```python
from build123d import *

# Parameters (mm, degrees)
SKETCH1_R               = 1.5
BOSS_EXTRUDE1_DEPTH     = 5
BOSS_EXTRUDE2_DEPTH     = 40
CUT_EXTRUDE1_DEPTH      = 91.434261951
BOSS_EXTRUDE3_START     = -5
BOSS_EXTRUDE3_OUTLINE_R = 2
BOSS_EXTRUDE3_DEPTH     = 5
CUT_EXTRUDE2_START      = -10
CUT_EXTRUDE2_DEPTH      = 10


# Read off the part's stored shape, not the designer's step: Boss-Extrude3
with BuildPart() as part:
    # Sketch1 → Boss-Extrude1 (new body)
    with BuildSketch(Plane(origin=(0, 0, 0), x_dir=(1, 0, 0), z_dir=(0, 1, 0))):
        with BuildLine():
            Line((-57.5, 45.38652637), (-44.5, -53.358277095))
            ThreePointArc((-44.5, -53.358277095), (0, -50.5), (44.5, -53.358277095))
            Line((44.5, -53.358277095), (57.5, 45.38652637))
            ThreePointArc((57.5, 45.38652637), (0, 51), (-57.5, 45.38652637))
        make_face()
        with Locations(Location((-5, 47.5, 0), (0, 0, 270))):
            Circle(SKETCH1_R, mode=Mode.SUBTRACT)
        with Locations(Location((-5, -47.5, 0), (0, 0, 270))):
            Circle(SKETCH1_R, mode=Mode.SUBTRACT)
        with Locations(Location((5, -47.5, 0), (0, 0, 90))):
            Circle(SKETCH1_R, mode=Mode.SUBTRACT)
        with Locations(Location((5, 47.5, 0), (0, 0, 90))):
            Circle(SKETCH1_R, mode=Mode.SUBTRACT)
    extrude(amount=BOSS_EXTRUDE1_DEPTH)

    # Sketch2 → Boss-Extrude2 (add)
    with BuildSketch(Plane(origin=(0, 5, 0), x_dir=(1, 0, 0), z_dir=(0, 1, 0))):
        with BuildLine():
            Line((-26.368366328, 19.603975201), (-20.985908119, -21.279853883))
            ThreePointArc((-20.985908119, -21.279853883), (-20.109118271, -22.872956361), (-18.384839881, -23.450537503))
            ThreePointArc((-18.384839881, -23.450537503), (0, -23), (18.384839881, -23.450537503))
            ThreePointArc((18.384839881, -23.450537503), (20.109118271, -22.872956361), (20.985908119, -21.279853883))
            Line((20.985908119, -21.279853883), (26.368366328, 19.603975201))
            ThreePointArc((26.368366328, 19.603975201), (25.841207036, 21.492926829), (24.11319073, 22.420285883))
            ThreePointArc((24.11319073, 22.420285883), (0, 23.5), (-24.11319073, 22.420285883))
            ThreePointArc((-24.11319073, 22.420285883), (-25.841207036, 21.492926829), (-26.368366328, 19.603975201))
        make_face()
    extrude(amount=BOSS_EXTRUDE2_DEPTH)

    # Sketch3 → Cut-Extrude1 (cut, through all)
    with BuildSketch(Plane(origin=(0, 0, 0), x_dir=(1, 0, 0), z_dir=(0, 1, 0))):
        with BuildLine():
            Line((-21.18897611, 19.181297446), (-16.295136113, -17.99110784))
            ThreePointArc((-16.295136113, -17.99110784), (0, -17.643611739), (16.295136113, -17.99110784))
            Line((16.295136113, -17.99110784), (21.18897611, 19.181297446))
            ThreePointArc((21.18897611, 19.181297446), (0, 19.717805469), (-21.18897611, 19.181297446))
        make_face()
    extrude(amount=CUT_EXTRUDE1_DEPTH, mode=Mode.SUBTRACT)

    # Boss-Extrude3 outline → Boss-Extrude3 (add)
    # profile 1 of 4: a face of its own
    with BuildSketch(Plane.XZ.offset(BOSS_EXTRUDE3_START)):
        with BuildLine():
            Line((-44.496886412, -57.390761561), (-40.51552272, -48.226360981))
            ThreePointArc((-40.51552272, -48.226360981), (-49.028326901, -46.92944202), (-57.5, -45.38652637))
            Line((-57.5, -45.38652637), (-55.934374164, -55.884987732))
            ThreePointArc((-55.934374164, -55.884987732), (-50.783157153, -60.948669168), (-44.496886412, -57.390761561))
        make_face()
        with Locations((-50, -55)):
            Circle(BOSS_EXTRUDE3_OUTLINE_R, mode=Mode.SUBTRACT)
    # profile 2 of 4: a face of its own
    with BuildSketch(Plane.XZ.offset(BOSS_EXTRUDE3_START)):
        with BuildLine():
            Line((40.51552272, -48.226360981), (44.496886412, -57.390761561))
            ThreePointArc((44.496886412, -57.390761561), (50.783157153, -60.948669168), (55.934374164, -55.884987732))
            Line((55.934374164, -55.884987732), (57.5, -45.38652637))
            ThreePointArc((57.5, -45.38652637), (49.028326901, -46.92944202), (40.51552272, -48.226360981))
        make_face()
        with Locations((50, -55)):
            Circle(BOSS_EXTRUDE3_OUTLINE_R, mode=Mode.SUBTRACT)
    # profile 3 of 4: a face of its own
    with BuildSketch(Plane.XZ.offset(BOSS_EXTRUDE3_START)):
        with BuildLine():
            Line((44.5, 53.358277095), (40.209954991, 58.740009651))
            ThreePointArc((40.209954991, 58.740009651), (34.735068112, 60.948669168), (30.018376627, 57.398262905))
            Line((30.018376627, 57.398262905), (27.484562868, 51.587560448))
            ThreePointArc((27.484562868, 51.587560448), (36.003169058, 52.368295779), (44.5, 53.358277095))
        make_face()
        with Locations((35.518225265, 55)):
            Circle(BOSS_EXTRUDE3_OUTLINE_R, mode=Mode.SUBTRACT)
    # profile 4 of 4: a face of its own
    with BuildSketch(Plane.XZ.offset(BOSS_EXTRUDE3_START)):
        with BuildLine():
            ThreePointArc((-44.5, 53.358277095), (-36.003169058, 52.368295779), (-27.484562868, 51.587560448))
            Line((-27.484562868, 51.587560448), (-30.018376627, 57.398262905))
            ThreePointArc((-30.018376627, 57.398262905), (-34.735068112, 60.948669168), (-40.209954991, 58.740009651))
            Line((-40.209954991, 58.740009651), (-44.5, 53.358277095))
        make_face()
        with Locations((-35.518225265, 55)):
            Circle(BOSS_EXTRUDE3_OUTLINE_R, mode=Mode.SUBTRACT)
    extrude(amount=BOSS_EXTRUDE3_DEPTH)

    # Sketch9 → Cut-Extrude2 (cut)
    with BuildSketch(Plane(origin=(0, 45, 0), x_dir=(1, 0, 0), z_dir=(0, 1, 0)).offset(CUT_EXTRUDE2_START)):
        with BuildLine():
            Line((17.602749325, -19.55074577), (22.887903449, 20.593985408))
            ThreePointArc((22.887903449, 20.593985408), (0, 21.217805469), (-22.887903449, 20.593985408))
            Line((-22.887903449, 20.593985408), (-17.602749325, -19.55074577))
            ThreePointArc((-17.602749325, -19.55074577), (0, -19.143611739), (17.602749325, -19.55074577))
        make_face()
        with BuildLine():
            Line((16.295136113, -17.99110784), (21.18897611, 19.181297446))
            ThreePointArc((21.18897611, 19.181297446), (0, 19.717805469), (-21.18897611, 19.181297446))
            Line((-21.18897611, 19.181297446), (-16.295136113, -17.99110784))
            ThreePointArc((-16.295136113, -17.99110784), (0, -17.643611739), (16.295136113, -17.99110784))
        make_face(mode=Mode.SUBTRACT)
    extrude(amount=CUT_EXTRUDE2_DEPTH, mode=Mode.SUBTRACT)


solid = part.part
```
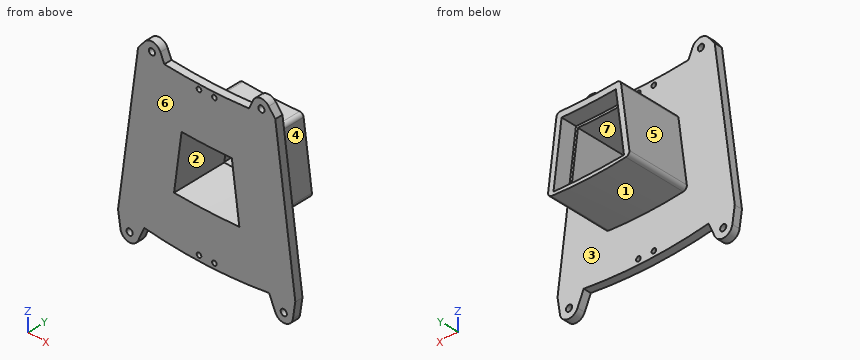
Model file for the job. Use its own axes, mm. Face numbers are marked on the shaded views. A direction names the side the tool comes from. Coordinates: 2 decimals unless noted, no trailing zeros. Loops run counter-clockwise (first coordinate to the right, second up) from the corner with the lowest first, then second, coordinate; pieces in that order, holes last. Notation, with made-up numbers: (40, -40) - (86, -40) arc R19 ccw to (86, -7) - close; hole circle Ø7 at (-10, 56.5). An arc over 180 degrees is marked (long way). Answer as a JSON object with one key per item and string values. Group by question number.
(1) Flat gauge pins, fed straight in: pin 1 (6.5 mm diameter, centred on x = 50, z = -55, fed in from -Y); pin 2 (1 mm diameter, centred on x = 32, z = -6, fed in from +Y); pin 3 (5 mm diameter, centred on x = -20.5, y = 6.5, fed in from -Z); pin 4 (6 mm diameter, centred on x = 9.5, y = 32, fed in from +Z). Where does each tip first touch, or does it go through?
(2) Probe line 1 along Z through (x, y) = (-1.5, 32); line 2 along X through (y, z) = (2.8, -47.5); line 3 along Y through (x, z) = (51, -44). List the from-to ranges inside material, lowest first.
(3) Two-plate mould, pull along Z, no slides. Class the marked faces 1, 2 and 3: released by +Z, released by -Z, zero draft, split by the parting line, or undercut.
(4) Tool access for the marked faces 4, 5, 6 and 7: list every direction of +Z, -Z, +X, -X, +Y, -Y with a clear straight run to the whole face (end or side of a thin tool).
(5) Cut at B-B (y = 21). Give the cut face in (x, z), then the cut area to 3 significant figures.
(6) Cut at C-C (z = 55). Give the cut face in (x, y).
(7) Cut at D-D (x = -50). Give the cut face in (y, z).
(8) Cut at A-A (x = -8). Give the cut face in (y, z).
Geometry says:
{
 "1": {"pin 1": "stops at y = 0", "pin 2": "stops at y = 5", "pin 3": "stops at z = -50.42", "pin 4": "stops at z = 23.21"},
 "2": {"line 1": "z = -23.5 to -19.72, 17.65 to 23", "line 2": "x = -57.18 to -6.5, -3.5 to 3.5, 6.5 to 57.18", "line 3": "y = 0 to 5"},
 "3": {"face 1": "released by -Z", "face 2": "undercut", "face 3": "zero draft"},
 "4": {"face 4": "+Z, +X, +Y", "face 5": "+Z, -X, +Y", "face 6": "+Z, -Z, +X, -X, -Y", "face 7": "+Y, -Y"},
 "5": {"outline": "(-26.37, -19.6) arc R2.5 ccw to (-24.11, -22.42) arc R269.8 ccw to (24.11, -22.42) arc R2.5 ccw to (26.37, -19.6) - (20.99, 21.28) arc R2.5 ccw to (18.38, 23.45) arc R375.34 cw to (-18.38, 23.45) arc R2.5 ccw to (-20.99, 21.28) - close; hole (-21.19, -19.18) arc R418.69 ccw to (21.19, -19.18) - (16.3, 17.99) arc R382.24 cw to (-16.3, 17.99) - close", "area": "793 mm^2"},
 "6": {"outline": "(-43.19, 0) - (-37.52, 0) - (-37.52, 5) - (-43.19, 5) - close; (-33.52, 0) - (-28.97, 0) - (-28.97, 5) - (-33.52, 5) - close; (28.97, 0) - (33.52, 0) - (33.52, 5) - (28.97, 5) - close; (37.52, 0) - (43.19, 0) - (43.19, 5) - (37.52, 5) - close"},
 "7": {"outline": "(0, -61) - (5, -61) - (5, -57) - (0, -57) - close; (0, -53) - (5, -53) - (5, 11.58) - (0, 11.58) - close"},
 "8": {"outline": "(0, -50.89) - (5, -50.89) - (5, -23.38) - (45, -23.38) - (45, -21.14) - (35, -21.14) - (35, -19.64) - (0, -19.64) - close; (0, 17.73) - (35, 17.73) - (35, 19.23) - (45, 19.23) - (45, 23.09) - (5, 23.09) - (5, 50.59) - (0, 50.59) - close"}
}
